Geometry: final body of the model. Coordinates: model frame, mm. Round coordinates to 2 decimals unless told otherwise and drop trailing zeros. Write each loop counter-clockwise with the first axis right and the second up, starting at its lowest first coordinate (ties: lowest second). Pieces come first, ordered by that corner, then holes. Notation, with made-up numbers: M 87,69.5 L 139,69.5 A20 ccw 139,91.5 Z; hole C 89.5,18.25 d10. An arc over 180 degrees is marked long. Use one line per item in the form item = value. Start each with the question number.
Item 1: Section query C-C (y = 0.3). Return loops of the section in (x, z) (3 decimals).
Item 2: Ray query, probe 1 along Z at (x, y) = (-52, 0.85) (3 decimals); probe 2 along X at (y, z) = (0.9, -2.5); probe 3 along X at (y, z) = (0.95, 0.75). Return the intervals inside material, ascending.
Item 3: Section query A-A (z = 0). Return loops of the section in (x, y) (1 decimal).
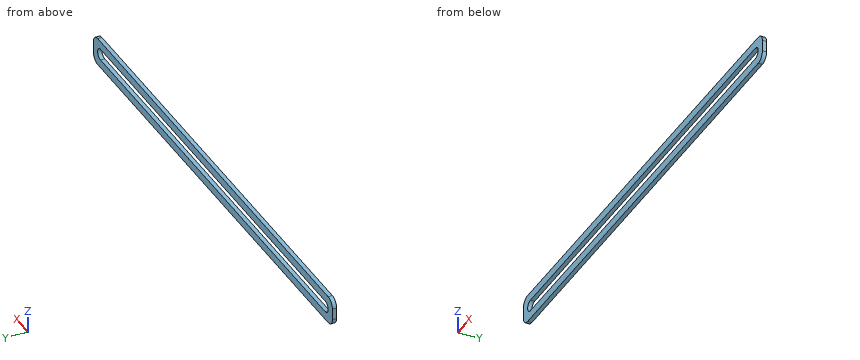
from build123d import *

# Parameters (mm, degrees)
SKETCH1_W           = 177.8
SKETCH1_H           = 10.65
BOSS_EXTRUDE1_DEPTH = 1.5875
FILLET1_R           = 3.175


with BuildPart() as part:
    # Sketch1 → Boss-Extrude1 (new body)
    with BuildSketch(Plane(origin=(0, 0, 0), x_dir=(1, 0, 0), z_dir=(0, 1, 0))):
        Rectangle(SKETCH1_W, SKETCH1_H)
        with BuildLine():
            Line((-83.575, 2.15), (83.575, 2.15))
            ThreePointArc((83.575, 2.15), (85.725, 0), (83.575, -2.15))
            Line((83.575, -2.15), (-83.575, -2.15))
            ThreePointArc((-83.575, -2.15), (-85.725, 0), (-83.575, 2.15))
        make_face(mode=Mode.SUBTRACT)
    extrude(amount=BOSS_EXTRUDE1_DEPTH)

    # Fillet1
    fillet1_edges = [part.edges().sort_by_distance(p)[0] for p in [
        (88.9, 0.79375, 5.325),
        (-88.9, 0.79375, 5.325),
        (-88.9, 0.79375, -5.325),
        (88.9, 0.79375, -5.325),
    ]]
    fillet(fillet1_edges, radius=FILLET1_R)


solid = part.part
Working result:
q1.outline = M -88.9,-2.15 A3.175 ccw -85.725,-5.325 L 85.725,-5.325 A3.175 ccw 88.9,-2.15 L 88.9,2.15 A3.175 ccw 85.725,5.325 L -85.725,5.325 A3.175 ccw -88.9,2.15 Z; hole M -83.575,-2.15 L 83.575,-2.15 A2.15 ccw 83.575,2.15 L -83.575,2.15 A2.15 ccw Z
q2.probe_1 = -5.325 to -2.15, 2.15 to 5.325
q2.probe_2 = -88.88 to 88.88
q2.probe_3 = -88.9 to -85.59, 85.59 to 88.9
q3.outline = M -88.9,0 L -85.7,0 L -85.7,1.6 L -88.9,1.6 Z; M 85.7,0 L 88.9,0 L 88.9,1.6 L 85.7,1.6 Z
